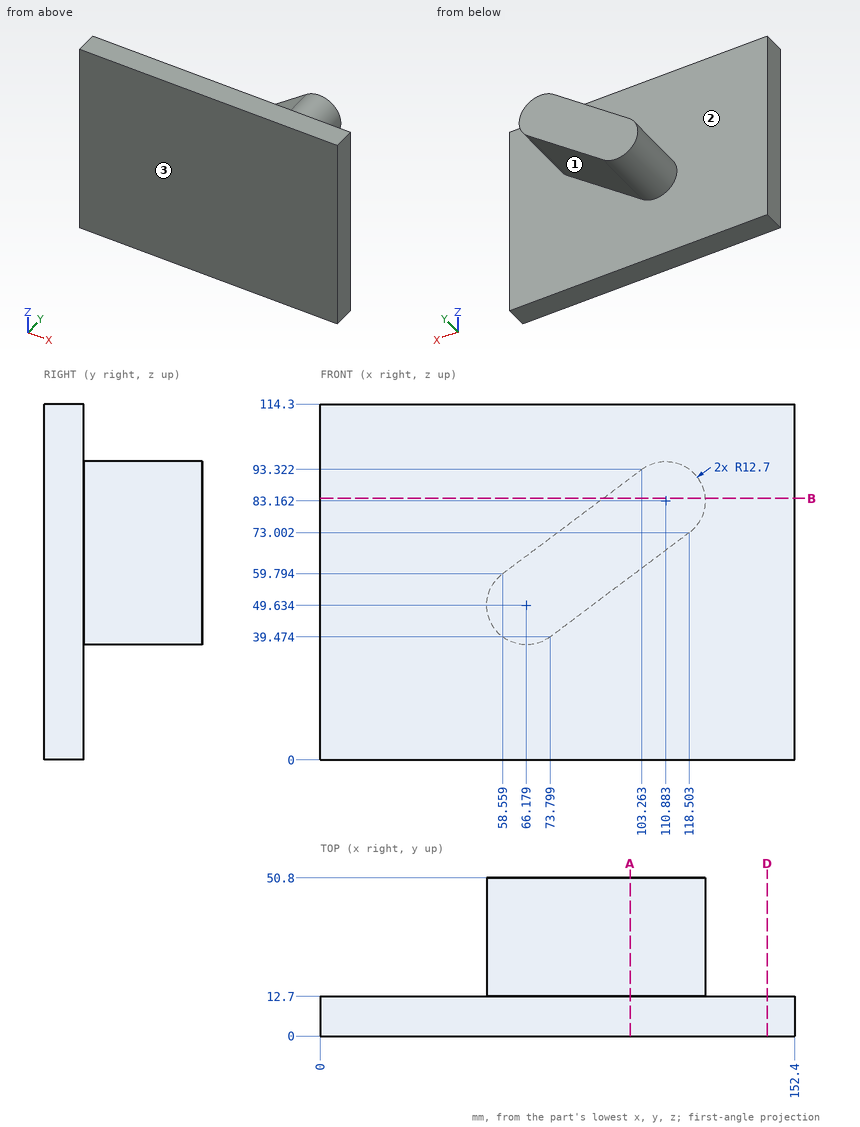
Part print with two shaded views. Sizes in mm from the minimum x, y, z corner. A direction names the side the tool comes from. Give positions to 0.01 mm unless a question says otherwise; leave off trailing zeros. Order: outer loops, then holes, each group sorted by start corner. A loop starts at its lowest first (then second) coordinate and runs counter-clockwise, first axis right, second up. Notation, with made-up numbers: M 63,4.25 L 104,4.25 A17 cw 104,30.25 Z; hole C 23.5,50.25 d11. An arc over 180 degrees is marked long. Write item = value, one per line.
Q1. Flat gauge pins, fed straight in: pin 1 (5 mm diameter, centred on x = 78, y = 43, fed in from +Z); pin 2 (4 mm diameter, centred on x = 90, y = 21.5, fed in from -Z) (1 decimal); pin 3 (2 mm diameter, centred on x = 57, z = 21.5, fed in from -Y). Where does each tip first touch, or does it go through?
Derived:
pin_1 = 76.25
pin_2 = 50.1
pin_3 = 0
Q2. Drill centre lines: line 1 (Y direction, x = 91, z = 20); line 2 (X direction, y = 26.5, z = 68.5) (1 decimal); line 3 (X direction, y = 23, z = 69) (1 decimal). Where is each one in solid material? Low to high. Write a range as [from, to].
Derived:
line_1 = [0, 12.7]
line_2 = [70.2, 112.5]
line_3 = [70.8, 113.2]
Q3. Tool access for the marked faces 1, 2 and 3: list every direction of +Z, -Z, +X, -X, +Y, -Y with a clear straight run to the whole face (end or side of a thin tool).
Derived:
face_1 = -Z, +X, +Y
face_2 = +Y
face_3 = +Z, -Z, +X, -X, -Y
Q4. Cut at A-A, the plane x = 99.5. List the corners of the cut face in (y, z).
Derived:
outline = M 0,0 L 12.7,0 L 12.7,58.75 L 50.8,58.75 L 50.8,90.5 L 12.7,90.5 L 12.7,114.3 L 0,114.3 Z
Q5. Cut at D-D, the plane x = 143.5. List the corners of the cut face in (y, z), then the cut area to 3 significant figures.
Derived:
outline = M 0,0 L 12.7,0 L 12.7,114.3 L 0,114.3 Z
area = 1,450 mm2
Q6. Cut at B-B, the plane z = 84. List the corners of the cut face in (x, y) (1 decimal).
Derived:
outline = M 0,0 L 152.4,0 L 152.4,12.7 L 123.6,12.7 L 123.6,50.8 L 90.8,50.8 L 90.8,12.7 L 0,12.7 Z
